from build123d import *

# Parameters (mm, degrees)
BOSS_EXTRUDE1_DEPTH            = 10
LPATTERN2_COUNT                = 8
LPATTERN2_PITCH                = 60
M8_TAPPED_HOLE2_D              = 6.8
F_6_8_6_8_DIAMETER_HOLE1_D     = 6.8
F_6_8_6_8_DIAMETER_HOLE1_DEPTH = 8.0000094
F_6_8_6_8_DIAMETER_HOLE1_TIP   = 2.042926105
M6_TAPPED_HOLE1_D              = 5


with BuildPart() as part:
    # Sketch1 → Boss-Extrude1 (new, symmetric)
    with BuildSketch(Plane(origin=(0, 0, 0), x_dir=(1, 0, 0), z_dir=(0, 1, 0))):
        with BuildLine():
            Line((0, 0), (496.825, 0))
            ThreePointArc((496.825, 0), (499.07006403, 0.92993597), (500, 3.175))
            Line((500, 3.175), (500, 46.825))
            ThreePointArc((500, 46.825), (499.07006403, 49.07006403), (496.825, 50))
            Line((496.825, 50), (70.2, 50))
            ThreePointArc((70.2, 50), (61.219743879, 53.719743879), (57.5, 62.7))
            Line((57.5, 62.7), (57.5, 146.825))
            ThreePointArc((57.5, 146.825), (56.57006403, 149.07006403), (54.325, 150))
            Line((54.325, 150), (0, 150))
            Line((0, 150), (0, 0))
        make_face()
    extrude(amount=BOSS_EXTRUDE1_DEPTH, both=True)

    # Sketch3 → M6 Tapped Hole2 (revolve, cut)
    with BuildSketch(Plane(origin=(45.5, 10, -25), x_dir=(0, 0, 1), z_dir=(1, 0, 0))):
        Polygon((0, 0), (0, 29.492951548), (2.5, 27.9908), (2.5, 0), align=None)
    m6_tapped_hole2 = revolve(axis=Axis((45.5, 16.35, -25), (0, -1, 0)), mode=Mode.SUBTRACT)

    # LPattern2: M6 Tapped Hole2 ×8
    with Locations(*[(i * LPATTERN2_PITCH, 0, 0) for i in range(1, LPATTERN2_COUNT)]):
        add(m6_tapped_hole2, mode=Mode.SUBTRACT)

    # M8 Tapped Hole2 (through all)
    with Locations(Plane(origin=(0, 10, 0), x_dir=(1, 0, 0), z_dir=(0, 1, 0))):
        with Locations((45.5, 131), (21.5, 131), (45.5, 71), (21.5, 71)):
            Hole(M8_TAPPED_HOLE2_D / 2)

    # Ø6.8 (6.8) Diameter Hole1
    with Locations(Plane(origin=(0, 10, 0), x_dir=(1, 0, 0), z_dir=(0, 1, 0))):
        with Locations((36.5, 140.950000036), (6.5, 140.950000036), (6.5, 40.950000036), (36.5, 40.950000036)):
            Hole(F_6_8_6_8_DIAMETER_HOLE1_D / 2, depth=F_6_8_6_8_DIAMETER_HOLE1_DEPTH)
            with Locations((0, 0, -(F_6_8_6_8_DIAMETER_HOLE1_DEPTH + F_6_8_6_8_DIAMETER_HOLE1_TIP / 2))):  # 118° drill point
                Cone(0, F_6_8_6_8_DIAMETER_HOLE1_D / 2, F_6_8_6_8_DIAMETER_HOLE1_TIP, mode=Mode.SUBTRACT)

    # M6 Tapped Hole1 (through all)
    with Locations(Plane(origin=(0, 10, 0), x_dir=(1, 0, 0), z_dir=(0, 1, 0))):
        with Locations((6.5, 140.950000036), (36.5, 140.950000036), (36.5, 40.950000036), (6.5, 40.950000036)):
            Hole(M6_TAPPED_HOLE1_D / 2)


solid = part.part
Input: part model. Units: mm. Frame: model coordinates. A direction names the side the tool comes from. Coordinates: 2 decimals unless noted, no trailing zeros. Order: outer loops, then holes, each group sorted by start corner. A loop starts at its lowest first (then second) coordinate and runs counter-clockwise, first axis right, second up. Notation, with made-up numbers: M 42,-20.75 L 49,-20.75 A19 cw 49,15.25 Z; hole C 72,10 d6. An arc over 180 degrees is marked long. Write item = value, one per line. Start each with the question number.
(1) Section C-C on x = 305.5. Output: boundary loops of the cut face in (y, z), and give its area (3 significant figures).
(2) Section B-B on z = -102.5. Output: boundary loops of the cut face in (x, y), and give its area (3 significant figures).
(3) Section A-A on y = -5.5. Give the number of separate pieces and of enclosed holes in the cut face, and give its area (3 significant figures).
(4) Line query: line 1 along Z through (x, y) = (45.5, 5.25); line 2 along X through (y, z) = (-4.25, -140.95); line 3 along Z through (x, y) = (6.5, 4.5). Output: solid intervals per line, ascending. Write a range as [from, to].
(5) Reachability of faces 1 (the flat face through (286, 0, -50)), 2 (the flat face through (28, 0, -150)) from +Z, -Z, +X, -X, +Y, -Y: full face, straight path, thin tool, end or side. Return the list, or none.
(6) First-contact query: P1, Ø1.5, axis at y = -2, z = -111.5, coming from the +X side; P2, Ø1, axis at y = -7, z = -120.5, coming from the -X side; P3, Ø6.5, axis at x = 6.5, z = -40.95, coming from the +Y side. Flat tips, straight axial feed; report the tip coordinate or a pass-through.
Result set:
q1.outline = M -10,-50 L 10,-50 L 10,0 L -10,0 Z
q1.area = 1,000 mm²
q2.outline = M 0,-10 L 57.5,-10 L 57.5,10 L 0,10 Z
q2.area = 1,150 mm²
q3.separate_pieces = 1
q3.enclosed_holes = 16
q3.area = 30,400 mm²
q4.line_1 = [-150, -134.4], [-127.6, -74.4], [-67.6, -27.5], [-22.5, 0]
q4.line_2 = [0, 4], [9, 34], [39, 57.5]
q4.line_3 = [-150, -144.35], [-137.55, -44.35], [-37.55, 0]
q5.face_1 = -Z, +X, +Y, -Y
q5.face_2 = -Z, +X, -X, +Y, -Y
q6.P1 = 57.5
q6.P2 = 0
q6.P3 = 1.91
